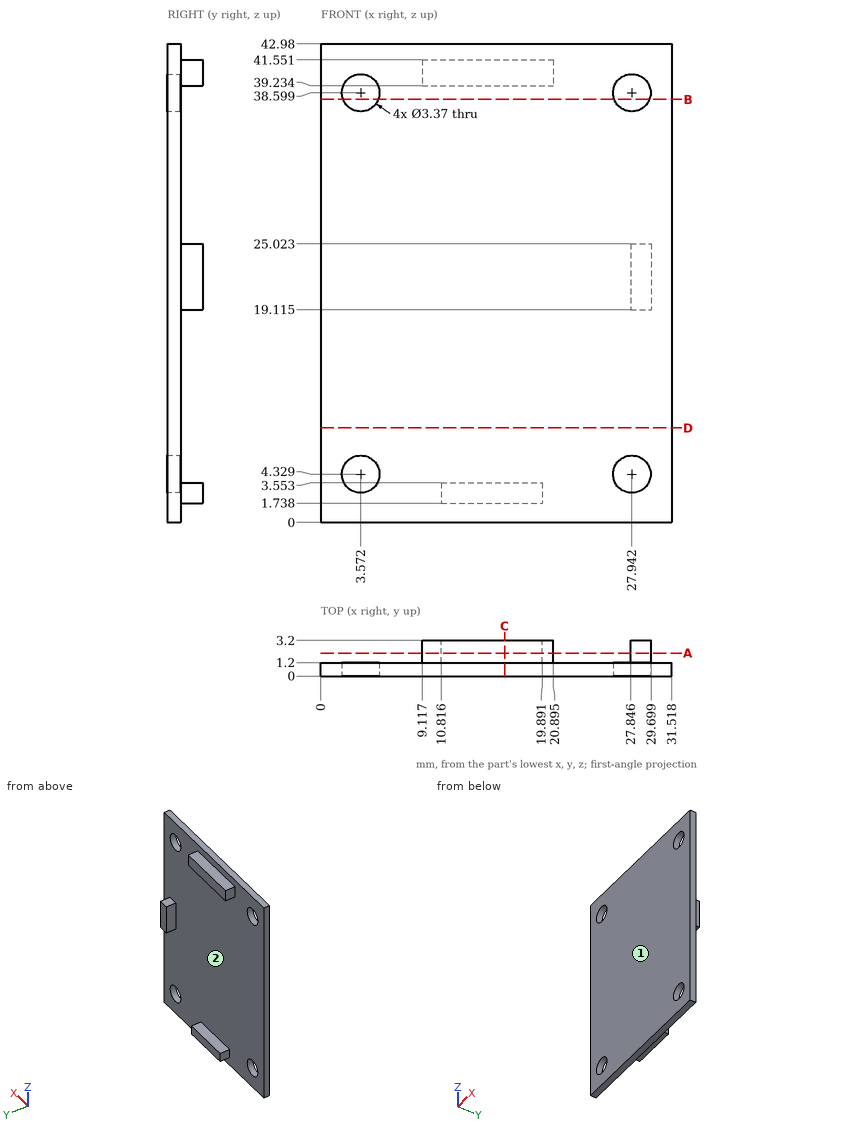
Check sheet for the drawn part. Datum: minimum x, y, z corner. Units: mm. Round coordinates to 2 decimals unless told otherwise and drop trailing zeros. Order: outer loops, then holes, each group sorted by start corner. A loop starts at its lowest first (then second) coordinate and runs counter-clockwise, first axis right, second up.
1) Mould release check, pull along Z, two halves, no side actions. Record for the marked faces 1 and 2: +Z half, -Z half, draft (parallel to the pull), parting line (faces both ways), or undercut.
2) Scan lines: line 1 (Z direction, x = 3.5, y = 0.65) (1 decimal); line 2 (Z direction, x = 18.5, y = 3); line 3 (X direction, y = 2.55, z = 20) (1 decimal). Record each from-to range of solid material in increasing order.
3) Section check D-D (z = 8.5). Record the boundary of the cut face in (x, y).
4) Section check A-A (y = 2.05). Give the number of separate pieces and of enclosed holes in the cut face.
5) Go/stop test with flat-tipped pins: pin 1 Ø1.6 at (y, z) = (2.5, 22) entering from +X; pin 2 Ø5 at (x, z) = (4.5, 8) entering from +Y; pin 3 Ø0.6 at (x, y) = (28.5, 2.5) entering from -Z (1 decimal). Record where each tip stops, or that it passes through.
6) Section check C-C (x = 16.5). Record the boundary of the cut face in (y, z).
7) Section check B-B (z = 38). Record the boundary of the cut face in (x, y).
Result:
1. face 1: draft
1. face 2: undercut
2. line 1: z = 0 to 2.6, 6 to 36.9, 40.3 to 43
2. line 2: z = 1.74 to 3.55, 39.23 to 41.55
2. line 3: x = 27.8 to 29.7
3. outline: (0, 0) - (31.52, 0) - (31.52, 1.2) - (0, 1.2) - close
4. separate pieces: 3
4. enclosed holes: 0
5. pin 1: stops at x = 29.7
5. pin 2: stops at y = 1.2
5. pin 3: stops at z = 19.1
6. outline: (0, 0) - (1.2, 0) - (1.2, 1.74) - (3.2, 1.74) - (3.2, 3.55) - (1.2, 3.55) - (1.2, 39.23) - (3.2, 39.23) - (3.2, 41.55) - (1.2, 41.55) - (1.2, 42.98) - (0, 42.98) - close
7. outline: (0, 0) - (2, 0) - (2, 1.2) - (0, 1.2) - close; (5.15, 0) - (26.37, 0) - (26.37, 1.2) - (5.15, 1.2) - close; (29.52, 0) - (31.52, 0) - (31.52, 1.2) - (29.52, 1.2) - close
